The drawing under review shows one solid part. Ordinate dimensions are in mm from its lowest x, y, z. A direction names the side the tool comes from. Coordinates: 2 decimals unless noted, no trailing zeros. Order: outer loops, then holes, each group sorted by start corner. A loop starts at its lowest first (then second) coordinate and runs counter-clockwise, first axis right, second up. Notation, with made-up numbers: (61, 4.5) -> (114, 4.5) arc R25 cw to (114, 26.5) -> close; hole circle Ø1 at (-7, -0.5). An arc over 180 degrees is marked (long way). Use one line per item in the form item = value.
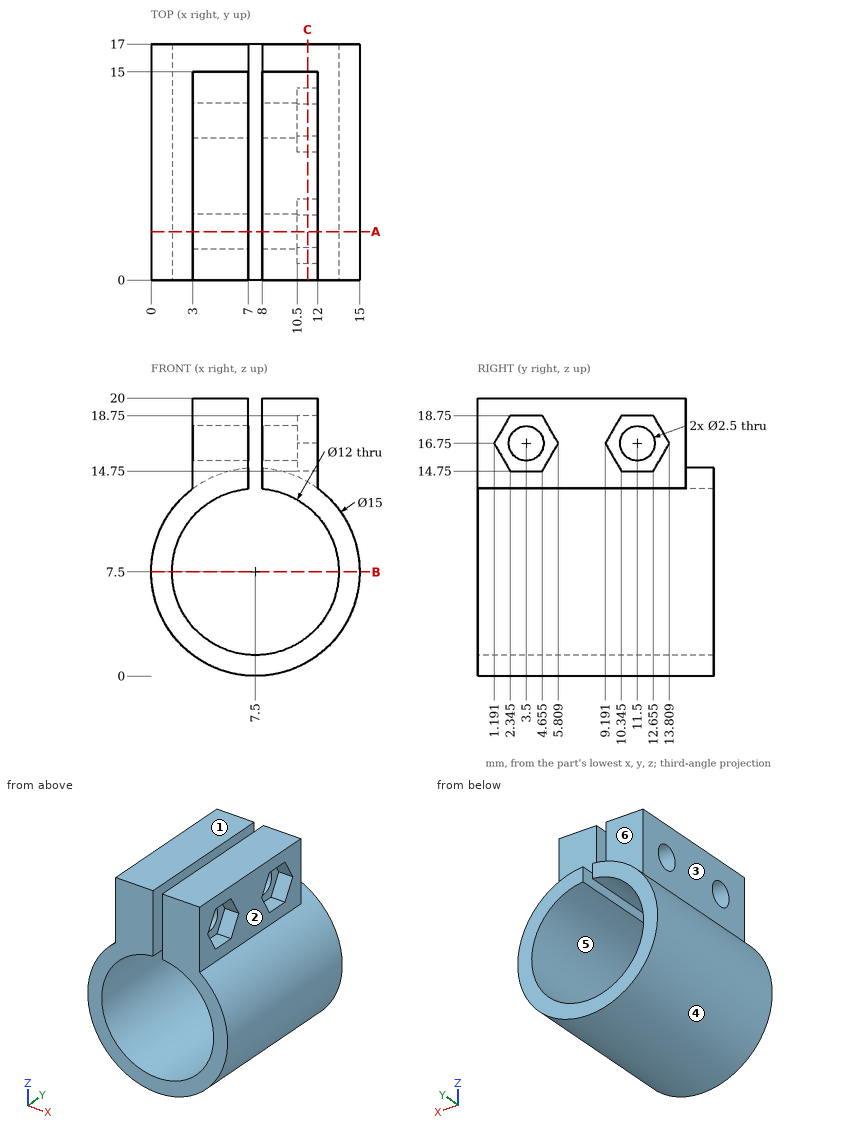
Item 1: We need section B-B (z = 7.5). Write out the cut boundary in (x, y).
Results found:
outline = (0, 0) -> (1.5, 0) -> (1.5, 17) -> (0, 17) -> close; (13.5, 0) -> (15, 0) -> (15, 17) -> (13.5, 17) -> close
Item 2: Draft analysis for pull direction X (two halves, no side actions). For the marked faces 4, 5 and 6, state which applies: released by +X, released by -X, zero draft, split by the parting line, or undercut.
Results found:
face_4 = split by the parting line
face_5 = undercut
face_6 = zero draft
Item 3: Tool access review of the marked faces 1, 2 and 3: name each direction out of +Z, -Z, +X, -X, +Y, -Y from which nothing blocks a thin tool from reaching the whole face with its end or side.
Results found:
face_1 = +Z, +X, -X, +Y, -Y
face_2 = +Z, +X, +Y, -Y
face_3 = +Z, -X, +Y, -Y
Item 4: To check wall thickness, follow L1, parallel to X at y = 8.25, z = 7.5; L2, parallel to Z at x = 5.7, y = 3.5; L3, parallel to X at y = 10.5, z = 15.25. State the ranges of each line that lie inside material, in increasing order. Write a range as from..to.
Results found:
L1 = 0..1.5, 13.5..15
L2 = 0.22..1.78, 13.22..15.5, 18..20
L3 = 3..7, 8..10.5
Item 5: We need section C-C (x = 11.25). State how many separate pieces and enclosed holes the cut face has, plus the area to 3 significant figures.
Results found:
separate_pieces = 2
enclosed_holes = 2
area = 124 mm²
Item 6: Clearance check with flat-ended pins moving along their axes: pin 1 (3 mm diameter, centred on x = 9, z = 15.5, fed in from +Y); pin 2 (0.8 mm diameter, centred on x = 11.5, y = 3.5, fed in from -Z); pin 3 (4 mm diameter, centred on y = 2.5, z = 14, fed in from +X); pin 4 (1.5 mm diameter, centred on y = 10, z = 4.5, fed in from -X) (1 decimal). State where each tip first meets the part, or that it passes through.
Results found:
pin_1 = 17
pin_2 = 0.92
pin_3 = 13.5
pin_4 = 0.3
Item 7: We need section A-A (y = 3.5). Write out the cut boundary in (x, z).
Results found:
outline = (3, 13.5) arc R7.5 ccw (long way) to (12, 13.5) -> (12, 14.75) -> (10.5, 14.75) -> (10.5, 15.5) -> (8, 15.5) -> (8, 13.48) arc R6 cw (long way) to (7, 13.48) -> (7, 15.5) -> (3, 15.5) -> close; (3, 18) -> (7, 18) -> (7, 20) -> (3, 20) -> close; (8, 18) -> (10.5, 18) -> (10.5, 18.75) -> (12, 18.75) -> (12, 20) -> (8, 20) -> close
